```python
from build123d import *

# Parameters (mm, degrees)
F0_W     = 135.431692
F0_H     = 102.052846
F1_DEPTH = 101.6
F3_DEPTH = 102.053845
F4_R     = 17.753754
F5_DEPTH = 135.432692


with BuildPart() as f1:
    # F0 (on Front) → F1 (new body)
    with BuildSketch(Plane.XZ):
        Rectangle(F0_W, F0_H)
    extrude(amount=F1_DEPTH)

    # F2 (on face) → F3 (cut, through all)
    with BuildSketch(Plane(origin=(0, 0, -51.026423), x_dir=(1, 0, 0), z_dir=(0, 0, -1))):
        Polygon((67.715846, 0), (67.715846, 101.6), (0, 101.6), align=None)
    extrude(amount=-F3_DEPTH, mode=Mode.SUBTRACT)

    # F4 (on face) → F5 (cut, through all)
    with BuildSketch(Plane(origin=(-67.715846, 0, 0), x_dir=(0, -1, 0), z_dir=(-1, 0, 0))):
        with Locations((44.151351, 0)):
            Circle(F4_R)
    extrude(amount=-F5_DEPTH, mode=Mode.SUBTRACT)


solid = f1.part
```
Geometry check sheet. Reference: the model listing, model coordinates, mm. Round coordinates to 2 decimals unless told otherwise and drop trailing zeros. Order: outer loops, then holes, each group sorted by start corner. A loop starts at its lowest first (then second) coordinate and runs counter-clockwise, first axis right, second up. Notation, with made-up numbers: (28.25, 16) - (47.25, 16) arc R23 cw to (47.25, 36) - close; hole circle Ø5 at (-10.5, -30). An arc over 180 degrees is marked (long way). Use a Markdown table: item, result. Add a question column.
1) Gauge pin test, flat ends, axial feed: P1, Ø1, axis at x = 20.5, z = 34.5, coming from the -Y side; P2, Ø1, axis at x = 44.5, z = -16, coming from the -Y side. Record the tip position at first contact, or that the pin passes through.
2) Thickness scan on line 1 along Y through (x, z) = (-39.5, 0); line 2 along Z through (x, y) = (22, -53); line 3 along Y through (x, z) = (12.5, 0). Record the ranges inside material, lowest first.
3) Section check C-C (x = -28.5). Record the cut outline in (y, z).
4) Section check A-A (y = -30). Record the cut outline in (x, z).
5) Mould release check, pull along Y, two halves, no side actions. Record for faces 1 (the flat face through (-34, -101.6, 1)), 2 (the flat face through (-16, -50, 51.026)), 3 (the flat face through (-1, 0, 1)), 4 (the cylindrical face through (-9.38, -26.415, 0.781)): released by +Y, released by -Y, zero draft, split by the parting line, or undercut.
6) Section check D-D (y = -68). Record the cut outline in (x, z), then the cut area to 3 significant figures.
7) Section check B-B (z = -16). Record the cut outline in (x, y), then the cut area to 3 significant figures.
Established:
| question | item | result |
|---|---|---|
| 1 | P1 | y = -71.59 |
| 1 | P2 | y = -35.58 |
| 2 | line 1 | -101.6 to -61.91, -26.4 to 0 |
| 2 | line 2 | -51.03 to -15.39, 15.39 to 51.03 |
| 2 | line 3 | -82.85 to -61.91, -26.4 to 0 |
| 3 | outline | (-101.6, -51.03) - (0, -51.03) - (0, 51.03) - (-101.6, 51.03) - close; hole circle Ø35.51 at (-44.15, 0) |
| 4 | outline | (-67.72, -51.03) - (47.72, -51.03) - (47.72, -10.72) - (-67.72, -10.72) - close; (-67.72, 10.72) - (47.72, 10.72) - (47.72, 51.03) - (-67.72, 51.03) - close |
| 5 | face 1 | released by -Y |
| 5 | face 2 | zero draft |
| 5 | face 3 | released by +Y |
| 5 | face 4 | undercut |
| 6 | outline | (-67.72, -51.03) - (22.39, -51.03) - (22.39, 51.03) - (-67.72, 51.03) - close |
| 6 | area | 9,200 mm2 |
| 7 | outline | (-67.72, -101.6) - (0, -101.6) - (33.16, -51.85) - (-67.72, -51.85) - close; (-67.72, -36.46) - (43.42, -36.46) - (67.72, 0) - (-67.72, 0) - close |
| 7 | area | 8,690 mm2 |
